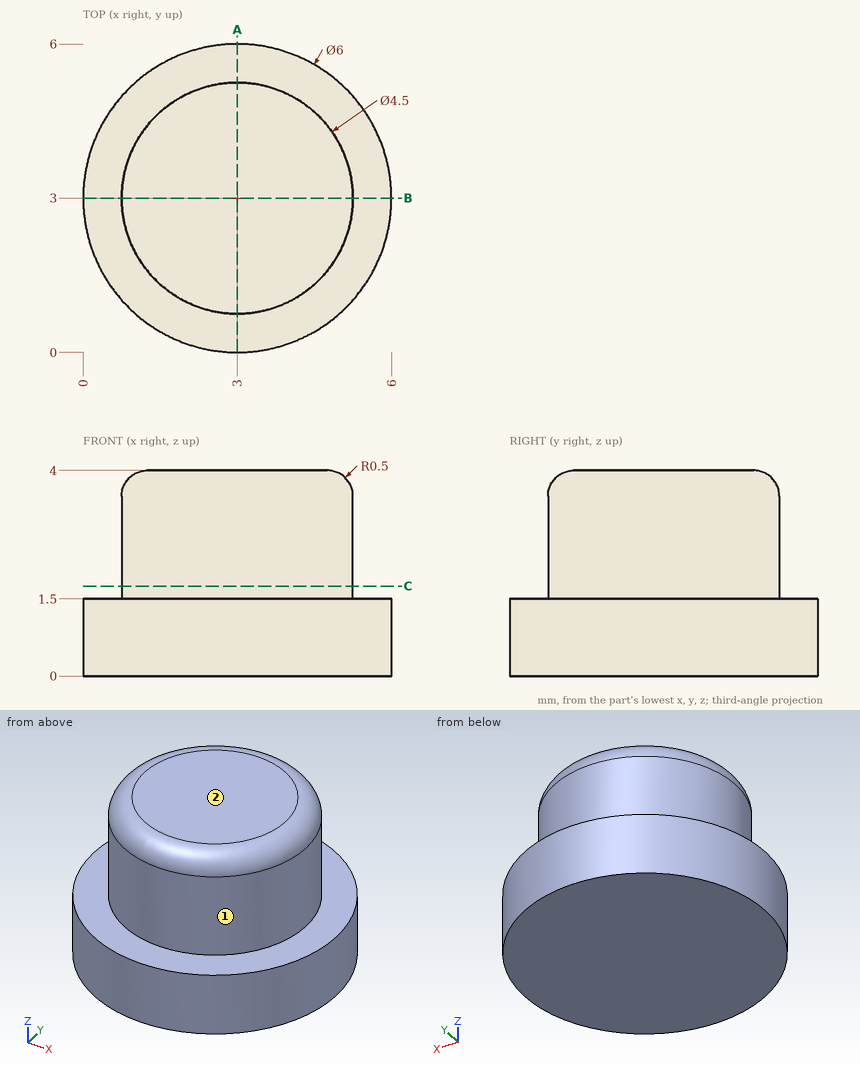
The figure shows three views and two pictorial views of one solid part (mm, origin at its lowest corner). Answer the questions. A direction names the side the tool comes from. Round coordinates to 2 decimals unless told otherwise and drop trailing zeros. Write each loop counter-clockwise with the first axis right and the second up, starting at its lowest first coordinate (ties: lowest second). Pieces come first, ordered by that corner, then holes. Notation, with made-up numbers: (19.25, 47.25) - (65.25, 47.25) arc R31 ccw to (65.25, 73.25) - close; hole circle Ø5 at (-17, 1). An arc over 180 degrees is marked (long way). Use one line per item in the form item = value. Start each with the question number.
Item 1: Find the intervals of material crossed by line 1 (Z direction, x = 3.55, y = 0.4); line 2 (X direction, y = 1.45, z = 2.5); line 3 (X direction, y = 4.1, z = 1.05), in increasing order. Write a range as [from, to].
Item 2: A tool of negligible diameter and unlimited length cuts with its end or side. For the marked faces 1 and 2, from which of +Z, -Z, +X, -X, +Y, -Y can it reach the whole face along a straight path? Write none if from no direction.
Item 3: A cutting plane is placed at A-A (x = 3). Write down the section's boundary in (y, z).
Item 4: A cutting plane is placed at C-C (z = 1.75). Write down the section's boundary in (x, y), plus the area to 3 significant figures.
Item 5: Flat-ended cylindrical pins translate along their axes: pin 1 Ø1.5 at (x, z) = (0.5, 1) entering from -Y; pin 2 Ø1.5 at (y, z) = (5, 1) entering from +X. Find the tip coordinate at first contact, or state that the pin passes through.
The answers:
q1.line_1 = [0, 1.5]
q1.line_2 = [1.37, 4.63]
q1.line_3 = [0.21, 5.79]
q2.face_1 = +Z
q2.face_2 = +Z, +X, -X, +Y, -Y
q3.outline = (0, 0) - (6, 0) - (6, 1.5) - (5.25, 1.5) - (5.25, 3.5) arc R0.5 ccw to (4.75, 4) - (1.25, 4) arc R0.5 ccw to (0.75, 3.5) - (0.75, 1.5) - (0, 1.5) - close
q4.outline = circle Ø4.5 at (3, 3)
q4.area = 15.9 mm^2
q5.pin_1 = 0.56
q5.pin_2 = 5.73
